from build123d import *

# Parameters (mm, degrees)
PAD_DEPTH       = 30
POCKET_DEPTH    = 30
POCKET001_DEPTH = 5
SKETCH012_R     = 3
POCKET002_DEPTH = 36.2220150744
SKETCH004_R     = 11.5
POCKET003_DEPTH = 2
SKETCH005_R     = 1.6
POCKET004_DEPTH = 5
SKETCH017_R     = 3
POCKET005_DEPTH = 48.8112135518
POCKET006_DEPTH = 48.8112135518
SKETCH019_W     = 5
SKETCH019_H     = 15
PAD001_DEPTH    = 15
POCKET007_DEPTH = 38.2766814448
FILLET_R        = 3
FILLET001_R     = 3
FILLET002_R     = 3
FILLET003_R     = 3
FILLET004_R     = 4
FILLET005_R     = 1


with BuildPart() as part:
    # Sketch → Pad (new body)
    with BuildSketch(Plane.XY):
        Polygon((-67, -15.6), (-67, -26.9528805906), (-13.1897864482, 37.175634728), (-67, 37.175634728), align=None)
    extrude(amount=PAD_DEPTH)

    # Sketch001 → Pocket (cut)
    with BuildSketch(Plane.XY.offset(30)):
        Polygon((-62, 32.175634728), (-62, -13.2154934933), (-23.9123210508, 32.175634728), align=None)
    extrude(amount=-POCKET_DEPTH, mode=Mode.SUBTRACT)

    # Sketch002 → Pocket001 (cut)
    with BuildSketch(Plane(origin=(-26.045511066, 21.8547787293, 0), x_dir=(0.6427876097, 0.7660444431, 0), z_dir=(0.7660444431, -0.6427876097, 0))):
        with BuildLine():
            ThreePointArc((7.9999570995, 17.5), (5.4999570995, 15), (7.9999570995, 12.5))
            Line((7.9999570995, 12.5), (11.9999570995, 12.5))
            ThreePointArc((11.9999570995, 12.5), (14.4999570995, 15), (11.9999570995, 17.5))
            Line((7.9999570995, 17.5), (11.9999570995, 17.5))
        make_face()
        with BuildLine():
            ThreePointArc((-20.0000429005, 17.5), (-22.5000429005, 15), (-20.0000429005, 12.5))
            Line((-20.0000429005, 12.5), (-16.0000429005, 12.5))
            ThreePointArc((-16.0000429005, 12.5), (-13.5000429005, 15), (-16.0000429005, 17.5))
            Line((-20.0000429005, 17.5), (-16.0000429005, 17.5))
        make_face()
    extrude(amount=-POCKET001_DEPTH, mode=Mode.SUBTRACT)

    # Sketch012 → Pocket002 (cut, through all)
    with BuildSketch(Plane(origin=(-29.8757332816, 25.0687167778, 0), x_dir=(-0.6427876097, -0.7660444431, 0), z_dir=(-0.7660444431, 0.6427876097, 0))):
        with Locations((20.0000429005, 15)):
            Circle(SKETCH012_R)
        with BuildLine():
            ThreePointArc((-11.9999570995, 19.5), (-16.4999570995, 15), (-11.9999570995, 10.5))
            Line((-11.9999570995, 10.5), (-7.9999570995, 10.5))
            ThreePointArc((-7.9999570995, 10.5), (-3.4999570995, 15), (-7.9999570995, 19.5))
            Line((-11.9999570995, 19.5), (-7.9999570995, 19.5))
        make_face()
    extrude(amount=POCKET002_DEPTH, mode=Mode.SUBTRACT)

    # Sketch004 → Pocket003 (cut)
    with BuildSketch(Plane(origin=(-67, 0, 0), x_dir=(0, -1, 0), z_dir=(-1, 0, 0))):
        with Locations((-1.4, 36)):
            Circle(SKETCH004_R)
    extrude(amount=-POCKET003_DEPTH, mode=Mode.SUBTRACT)

    # Sketch005 → Pocket004 (cut)
    with BuildSketch(Plane(origin=(-67, 0, 0), x_dir=(0, -1, 0), z_dir=(-1, 0, 0))):
        with Locations((-17.4, 20)):
            Circle(SKETCH005_R)
        with Locations((14.6, 20)):
            Circle(SKETCH005_R)
    extrude(amount=-POCKET004_DEPTH, mode=Mode.SUBTRACT)

    # Sketch017 → Pocket005 (cut, through all)
    with BuildSketch(Plane.YZ.offset(-62)):
        with Locations((-14.6, 20)):
            Circle(SKETCH017_R)
        with Locations((17.4, 20)):
            Circle(SKETCH017_R)
    extrude(amount=POCKET005_DEPTH, mode=Mode.SUBTRACT)

    # Sketch018 → Pocket006 (cut, through all)
    with BuildSketch(Plane.YZ.offset(-62)):
        with BuildLine():
            ThreePointArc((1.4000345084, 20), (16.63877916, 40.8764341185), (-7.88883473, 49.02756882))
            Line((-48.5999654916, 20), (-7.88883473, 49.02756882))
            Line((1.4000345084, 20), (-48.5999654916, 20))
        make_face()
    extrude(amount=POCKET006_DEPTH, mode=Mode.SUBTRACT)

    # Sketch019 → Pad001 (new body)
    with BuildSketch(Plane(origin=(-67, 0, 0), x_dir=(0, -1, 0), z_dir=(-1, 0, 0))):
        with Locations((-1.3999532833, 7.5)):
            Rectangle(SKETCH019_W, SKETCH019_H)
    extrude(amount=PAD001_DEPTH)

    # Sketch020 → Pocket007 (cut, through all)
    with BuildSketch(Plane.XZ.offset(1.1000467167)):
        Polygon((-82, 15), (-82, 0), (-67, 0), align=None)
    extrude(amount=-POCKET007_DEPTH, mode=Mode.SUBTRACT)

    # Fillet
    fillet_edges = [part.edges().sort_by_distance(p)[0] for p in [
        (-67, -26.952881, 15),
    ]]
    fillet(fillet_edges, radius=FILLET_R)

    # Fillet001
    fillet001_edges = [part.edges().sort_by_distance(p)[0] for p in [
        (-67, 37.175635, 15),
    ]]
    fillet(fillet001_edges, radius=FILLET001_R)

    # Fillet002
    fillet002_edges = [part.edges().sort_by_distance(p)[0] for p in [
        (-62, 32.175635, 15),
    ]]
    fillet(fillet002_edges, radius=FILLET002_R)

    # Fillet003
    fillet003_edges = [part.edges().sort_by_distance(p)[0] for p in [
        (-60.576001, -17.6, 20),
        (-57.380922, -11.6, 20),
        (-34.026768, 16.232397, 30),
    ]]
    fillet(fillet003_edges, radius=FILLET003_R)

    # Fillet004
    fillet004_edges = [part.edges().sort_by_distance(p)[0] for p in [
        (-67, -1.100047, 7.5),
        (-67, 3.899953, 7.5),
    ]]
    fillet(fillet004_edges, radius=FILLET004_R)

    # Fillet005
    fillet005_edges = [part.edges().sort_by_distance(p)[0] for p in [
        (-13.189786, 37.175635, 15),
    ]]
    fillet(fillet005_edges, radius=FILLET005_R)


solid = part.part
Can you work these out from the model? Positions are in its coordinate system, mm. A direction names the side the tool comes from. Coordinates: 2 decimals unless noted, no trailing zeros. Write each loop counter-clockwise with the first axis right and the second up, starting at its lowest first coordinate (ties: lowest second). Pieces come first, ordered by that corner, then holes. Notation, with made-up numbers: (73.5, 76) - (125.5, 76) arc R31 ccw to (125.5, 109) - close; hole circle Ø4 at (51.5, 40.5). An arc over 180 degrees is marked (long way). Return JSON: item names as keys, results as strings. Group by question number.
Item 1: If we section it at A-A (x = -56.5): Write out the boundary of the cut face in (y, z), then the cut area to 3 significant figures.
Item 2: We'd pull the mould along Y, two halves only. Please class faces 1 (the face through (-38.465, 7.054, 11.457)), 2 (the face through (-66.1, 36.32, 15.21)), 3 (the face through (-64.54, -15.46, 21.35)): pulls with the +Y half, pulls with the -Y half, needs draft (parallel to the pull), parting line crosses it, or undercut.
Item 3: Please list where these lines run through material, in increasing order: probe 1 along Z at (x, y) = (-65.25, 17.4); probe 2 along X at (y, z) = (14, 23); probe 3 along X at (y, z) = (-2, 3.5).
Item 4: Which directions (+Z, -Z, +X, -X, +Y, -Y) give clear straight access to the entire face, cutting with the end or side of a thin tool? Please do faces 4 (the face through (-34.87, 33.83, 14.9)), 5 (the face through (-41, 32.176, 15)), 6 (the face through (-65, 2, 28)).
Item 5: I'm going to push flat-ended pins straight in: pin 1 Ø3.5 at (y, z) = (17.4, 20) entering from +X; pin 2 Ø5.5 at (x, z) = (-77.5, 10.5) entering from +Y; pin 3 Ø0.8 at (x, y) = (-61.5, -20) entering from +Z. Where does each tip first touch, or does it pass through?
Item 6: If we section it at B-B (y = -14.6): Write out the boundary of the cut face in (x, z), then the cut area to 3 significant figures.
Return value:
{
 "1": {"outline": "(-14.44, 0) - (-6.66, 0) - (-6.66, 20) - (-9.4, 20) arc R3 ccw to (-12, 18.5) arc R3 cw to (-14.44, 17) - close; (32.18, 0) - (37.18, 0) - (37.18, 30) - (32.18, 30) - close", "area": "298 mm^2"},
 "2": {"face 1": "pulls with the -Y half", "face 2": "pulls with the +Y half", "face 3": "undercut"},
 "3": {"probe 1": "z = 0 to 18.4, 21.6 to 30", "probe 2": "x = -67 to -62, -39.16 to -32.64", "probe 3": "x = -68.47 to -62, -52.59 to -46.06"},
 "4": {"face 4": "+Y", "face 5": "+Z, -Z", "face 6": "+Z, -X"},
 "5": {"pin 1": "stops at x = -62", "pin 2": "stops at y = 3.9", "pin 3": "stops at z = 20"},
 "6": {"outline": "(-67, 0) - (-56.63, 0) - (-56.63, 17) - (-62, 17) - (-62, 18.4) - (-67, 18.4) - close; (-67, 21.6) - (-62, 21.6) - (-62, 30) - (-67, 30) - close", "area": "225 mm^2"}
}
